CAD build for the part. Positions are in the model's coordinates, mm. Face numbers are marked on the shaded views. A direction names the side the tool comes from. Coordinates: 2 decimals unless noted, no trailing zeros. Write each loop counter-clockwise with the first axis right and the second up, starting at its lowest first coordinate (ties: lowest second). Pieces come first, ordered by that corner, then holes. Notation, with made-up numbers: (59.25, 22) - (104.25, 22) arc R23 ccw to (104.25, 40) - close; hole circle Ø9 at (61, 80). An arc over 180 degrees is marked (long way). Answer in a Markdown table with one row per item. Add a question column.
Q1. Drill centre lines: line 1 along Y through (x, z) = (49, -28.5); line 2 along Z through (x, y) = (29, 1.35); line 3 along X through (y, z) = (1.5, 4.5). Where is each one in solid material? Low to high. Write a range as from..to.
Q2. Band-saw the part on A-A (x = 28). List the corners of the cut face in (y, z), and give its area (3 significant figures).
Q3. 3-axis set-ups, long thin cutter, end or side, ignore diameter. For the marked faces 1 and 2: which of +Z, -Z, +X, -X, +Y, -Y reach the whole face in a straight line?
Q4. Pin check, flat tips, straight feed: pin 1 (1.5 mm diameter, centred on y = 1, z = -15.5, fed in from +X); pin 2 (8 mm diameter, centred on x = -49, z = -12.5, fed in from -Y); pin 3 (0.9 mm diameter, centred on x = -24.5, y = 3, fed in from +Z). Stop position of each tip, or through.
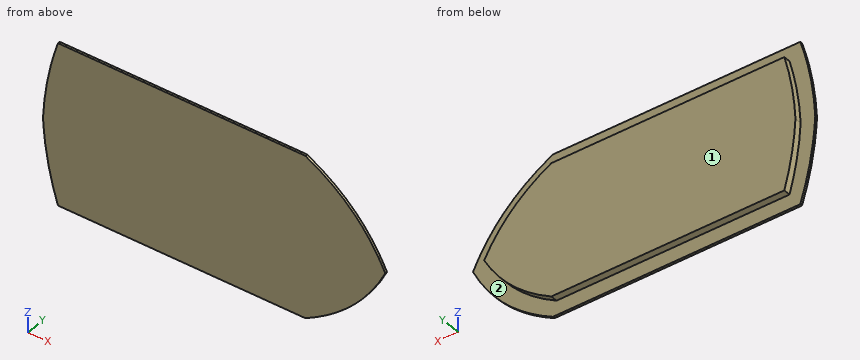
```python
from build123d import *

# Parameters (mm, degrees)
SALIENTE_EXTRUIR4_DEPTH = 1
SALIENTE_EXTRUIR5_DEPTH = 4


with BuildPart() as part:
    # Croquis1 → Saliente-Extruir4 (new body)
    with BuildSketch(Plane(origin=(0, 0, 0), x_dir=(1, 0, 0), z_dir=(0, 1, 0))):
        with BuildLine():
            Line((-68.807549393, -35.735609902), (38.825281278, -35.735609902))
            add(Edge.make_bspline(
                [(38.825281278, -35.735609902), (38.857624552, -35.718822416), (38.889937105, -35.702026903), (40.163492425, -35.039106907), (41.363053394, -34.379508835), (44.879608288, -32.340972971), (47.103940203, -30.908125592), (53.416675645, -26.4056608), (57.158292578, -23.128173527), (63.889280185, -15.928414127), (66.879657947, -12.004947025), (70.871982915, -5.502682168), (72.121484201, -3.228479298), (73.380247303, -0.652201666), (73.473116384, -0.460315749), (73.565425725, -0.267750564)],
                knots=[0.132682558, 0.132682558, 0.132682558, 0.132682558, 0.13425238, 0.13425238, 0.194615488, 0.194615488, 0.315341705, 0.315341705, 0.556794137, 0.556794137, 0.79824657, 0.79824657, 0.918972787, 0.918972787, 0.928652581, 0.928652581, 0.928652581, 0.928652581], degree=3))
            add(Edge.make_bspline(
                [(73.565425725, -0.267750564), (73.473116384, -0.07518538), (73.380247303, 0.116700538), (72.121484201, 2.692978169), (70.871982915, 4.967181039), (66.879657947, 11.469445896), (63.889280185, 15.392912998), (57.158292578, 22.592672399), (53.416675646, 25.870159671), (47.103940203, 30.372624464), (44.879608287, 31.805471842), (41.363053394, 33.844007706), (40.163492425, 34.503605779), (38.889937105, 35.166525774), (38.857624552, 35.183321288), (38.825281278, 35.200108773)],
                knots=[0.132682558, 0.132682558, 0.132682558, 0.132682558, 0.142362352, 0.142362352, 0.263088569, 0.263088569, 0.504541001, 0.504541001, 0.745993434, 0.745993434, 0.866719651, 0.866719651, 0.927082759, 0.927082759, 0.928652581, 0.928652581, 0.928652581, 0.928652581], degree=3))
            Line((38.825281278, 35.200108773), (-68.807549393, 35.200108773))
            add(Edge.make_bspline(
                [(-68.807549393, 35.200108773), (-70.080284046, 31.302990951), (-71.169252334, 27.374853959), (-72.991045883, 19.413196683), (-73.721201284, 15.377083685), (-74.541341264, 9.255508785), (-74.768651118, 7.205452815), (-75.107581304, 3.346349854), (-75.230698844, 1.538874232), (-75.318593087, -0.267750565)],
                knots=[0.290505717, 0.290505717, 0.290505717, 0.290505717, 0.524524567, 0.524524567, 0.760550999, 0.760550999, 0.878564216, 0.878564216, 0.980861336, 0.980861336, 0.980861336, 0.980861336], degree=3))
            add(Edge.make_bspline(
                [(-75.318593087, -0.267750565), (-75.230698844, -2.074375361), (-75.107581304, -3.881850983), (-74.768651118, -7.740953944), (-74.541341264, -9.791009913), (-73.721201284, -15.912584814), (-72.991045883, -19.948697811), (-71.169252334, -27.910355088), (-70.080284046, -31.838492079), (-68.807549393, -35.735609902)],
                knots=[0.290505717, 0.290505717, 0.290505717, 0.290505717, 0.392802838, 0.392802838, 0.510816054, 0.510816054, 0.746842486, 0.746842486, 0.980861336, 0.980861336, 0.980861336, 0.980861336], degree=3))
        make_face()
    extrude(amount=SALIENTE_EXTRUIR4_DEPTH)

    # Croquis4 → Saliente-Extruir5 (add)
    with BuildSketch(Plane(origin=(0, 0, 0), x_dir=(1, 0, 0), z_dir=(0, 1, 0))):
        with BuildLine():
            Line((37.247663382, 28.855017698), (-64.119969997, 28.855017698))
            add(Edge.make_bspline(
                [(-64.119969997, 28.855017698), (-65.485825703, 24.110871923), (-66.573936798, 19.303338214), (-68.190809552, 9.563299345), (-68.714330818, 4.66248528), (-68.96563874, -0.267750565)],
                knots=[0, 0, 0, 0, 0.5, 0.5, 1, 1, 1, 1], degree=3))
            add(Edge.make_bspline(
                [(-64.119969997, -29.390518826), (-65.485825703, -24.646373051), (-66.573936798, -19.838839342), (-68.190809552, -10.098800474), (-68.714330818, -5.197986409), (-68.96563874, -0.267750565)],
                knots=[0, 0, 0, 0, 0.5, 0.5, 1, 1, 1, 1], degree=3))
            Line((-64.119969997, -29.390518826), (37.247663382, -29.390518826))
            add(Edge.make_bspline(
                [(66.462106503, -0.267750564), (64.818621385, -3.374433842), (62.975742409, -6.335483667), (59.886080558, -10.539433832), (58.80173399, -11.900974536), (57.091612362, -13.882224457), (56.507662174, -14.532481759), (55.311926642, -15.812666099), (54.698983392, -16.443734837), (51.578159003, -19.532591798), (48.914439134, -21.777803713), (43.292419218, -25.869940939), (40.335081649, -27.71816757), (37.247663382, -29.390518826)],
                knots=[0, 0, 0, 0, 0.25, 0.25, 0.375, 0.375, 0.4375, 0.4375, 0.5, 0.5, 0.75, 0.75, 1, 1, 1, 1], degree=3))
            add(Edge.make_bspline(
                [(66.462106503, -0.267750564), (64.818621385, 2.838932714), (62.975742409, 5.799982539), (59.886080558, 10.003932703), (58.80173399, 11.365473408), (57.091612362, 13.346723328), (56.507662174, 13.996980631), (55.311926642, 15.277164971), (54.698983392, 15.908233708), (51.578159003, 18.99709067), (48.914439134, 21.242302584), (43.292419218, 25.334439811), (40.335081649, 27.182666442), (37.247663382, 28.855017698)],
                knots=[0, 0, 0, 0, 0.25, 0.25, 0.375, 0.375, 0.4375, 0.4375, 0.5, 0.5, 0.75, 0.75, 1, 1, 1, 1], degree=3))
        make_face()
    extrude(amount=SALIENTE_EXTRUIR5_DEPTH)


solid = part.part
```
Checked values:
| question | item | result |
|---|---|---|
| 1 | line 1 | y = 0..1 |
| 1 | line 2 | z = -28.86..29.39 |
| 1 | line 3 | x = -68.68..64.04 |
| 2 | outline | (0, -35.2) - (1, -35.2) - (1, -28.86) - (4, -28.86) - (4, 29.39) - (1, 29.39) - (1, 35.74) - (0, 35.74) - close |
| 2 | area | 246 mm² |
| 3 | face 1 | +Z, -Z, +X, -X, +Y |
| 3 | face 2 | +Y |
| 4 | pin 1 | stops at x = 64.2 |
| 4 | pin 2 | stops at y = 0 |
| 4 | pin 3 | stops at z = 29.39 |
